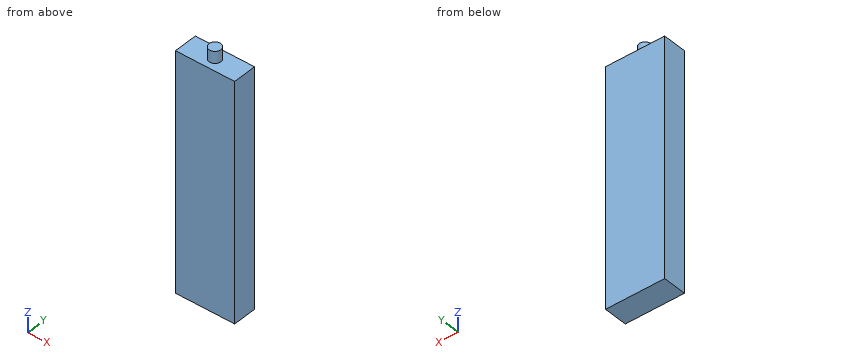
from build123d import *

# Parameters (mm, degrees)
SKETCH_1_W      = 50
SKETCH_1_H      = 200
EXTRUDE_1_DEPTH = 10
SKETCH_2_R      = 5
EXTRUDE_2_DEPTH = 10


with BuildPart() as part:
    # 草图1 → 凸台-拉伸1 (new body, symmetric)
    with BuildSketch(Plane(origin=(0, 0, 0), x_dir=(1, 0, 0), z_dir=(0, 1, 0))):
        with Locations((25, -100)):
            Rectangle(SKETCH_1_W, SKETCH_1_H)
    extrude(amount=EXTRUDE_1_DEPTH, both=True)

    # 草图2 → 凸台-拉伸2 (add, symmetric)
    with BuildSketch(Plane.XY.offset(200)):
        with Locations((25, 0)):
            Circle(SKETCH_2_R)
    extrude(amount=EXTRUDE_2_DEPTH, both=True)


solid = part.part
Geometry: final body of the model. Coordinates: model frame, mm. Give positions to 0.01 mm unless a question says otherwise; leave off trailing zeros. Write each loop counter-clockwise with the first axis right and the second up, starting at its lowest first coordinate (ties: lowest second). Pieces come first, ordered by that corner, then holes. Notation, with made-up numbers: (32, -10) -> (84, -10) arc R33 cw to (84, 20) -> close; hole circle Ø2 at (-36.5, 9). An arc over 180 degrees is marked (long way). Answer in a Markdown table with one row per item.
(1) Section query A-A on y = 0. Return loops of the section in (x, z), then the cut area to 3 significant figures.
Answers below:
| item | result |
|---|---|
| outline | (0, 0) -> (50, 0) -> (50, 200) -> (30, 200) -> (30, 210) -> (20, 210) -> (20, 200) -> (0, 200) -> close |
| area | 10,100 mm^2 |
(2) Section query B-B on x = 25. Return loops of the section in (y, z).
Answers below:
| item | result |
|---|---|
| outline | (-10, 0) -> (10, 0) -> (10, 200) -> (5, 200) -> (5, 210) -> (-5, 210) -> (-5, 200) -> (-10, 200) -> close |
(3) Section query C-C on x = 14. Return loops of the section in (y, z), then the cut area to 3 significant figures.
Answers below:
| item | result |
|---|---|
| outline | (-10, 0) -> (10, 0) -> (10, 200) -> (-10, 200) -> close |
| area | 4,000 mm^2 |
(4) Pin query (flat end, axial travel): pin 1 (2 mm diameter, centred on x = 24, y = 6.5, fed in from -Z); pin 2 (1.5 mm diameter, centred on x = 8, y = 1.5, fed in from +Z). Return the tip coordinate at first contact, or that it passes through.
Answers below:
| item | result |
|---|---|
| pin 1 | z = 0 |
| pin 2 | z = 200 |
(5) Ray query, line 1 along Z through (x, y) = (36, 3). Return the intervals inside material, ascending. Write a range as [from, to].
Answers below:
| item | result |
|---|---|
| line 1 | [0, 200] |
